Design review of the part built by this model. Coordinates are the model's own, in mm. A direction names the side the tool comes from. Round coordinates to 2 decimals unless told otherwise and drop trailing zeros. Order: outer loops, then holes, each group sorted by start corner. A loop starts at its lowest first (then second) coordinate and runs counter-clockwise, first axis right, second up. Notation, with made-up numbers: M 2.25,-25.5 L 53.25,-25.5 A13 cw 53.25,-21.5 Z; hole C -25,39 d8. An arc over 180 degrees is marked long. Use a Markdown table: item, result. Add a question column.
(1) Take a section at D-D (x = -2.75). Write out the cut boundary in (y, z), then the cut area to 3 significant figures.
(2) Take a section at A-A (z = -80.75). Write out the cut boundary in (x, y).
(3) The part is to be moulded in two halves that separate along X. For faces 1 (the face through (-0.212, -5.865, -82.733)), 2 (the face through (0, 3, -79.691)), 3 (the face through (5.18, 3.06, -82.73)), 4 (the face through (-6.454, -2.814, -94.712)), say which applies: released by +X, released by -X, zero draft, split by the parting line, or undercut.
(4) Take a section at C-C (x = 0). Write out the cut boundary in (y, z).
(5) For pin 1 (1 mm diameter, centred on x = -5.5, z = -92.5, fed in from +Y); pin 2 (1 mm diameter, centred on y = 1.5, z = -84.5, fed in from -X); pin 3 (6 mm diameter, centred on x = -3, z = -82.5, fed in from +Y), all flat-tipped, find the tip position at first contact; note any pin that passes through.
(6) Take a section at B-B (y = 0). Write out the cut boundary in (x, z), then the cut area to 3 significant figures.
(7) To check wall thickness, follow probe 1 along Z at (x, y) = (0.75, -8.5); probe 2 along Z at (x, y) = (-6.25, -0.75); probe 3 along Y at (x, z) = (5.25, -93.5). State the ranges of each line that lie inside material, in increasing order. Write a range as from..to.
(8) Machinability: for faces 5 (the face through (0.9, 2, -82.7)), 6 (the face through (3.94, -2.81, -94.71)), 7 (the face through (-0.2, -6.1, -85.691)), 8 (the face through (-0.018, 4.034, -82.733)), 9 (the face through (-3.408, -3.633, -91.959)), which of the approach directions +Z, -Z, +X, -X, +Y, -Y give a long, thin tool a straight path to every point of the face, cutting with its end or side? Answer none if there is none.
```python
from build123d import *

# Parameters (mm, degrees)
SKETCH2_R           = 10
SKETCH2_R_2         = 2.1
SKETCH2_R_3         = 1.2
BOSS_EXTRUDE1_DEPTH = 3
SKETCH3_R           = 10
SKETCH3_R_2         = 2
SKETCH3_R_3         = 2.1
BOSS_EXTRUDE2_DEPTH = 2.5
SKETCH4_R           = 2.1
BOSS_EXTRUDE3_DEPTH = 5
FILLET1_R           = 0.8
SKETCH5_R           = 2.1
BOSS_EXTRUDE4_DEPTH = 6


with BuildPart() as part:
    # Sketch2 → Boss-Extrude1 (new body)
    with BuildSketch(Plane.XY.offset(-96.191169136)):
        Circle(SKETCH2_R)
        Circle(SKETCH2_R_2, mode=Mode.SUBTRACT)
        with Locations((-0.05897353, 6.133133301)):
            Circle(SKETCH2_R_3, mode=Mode.SUBTRACT)
        with Locations((5.137178892, -2.866866699)):
            Circle(SKETCH2_R_3, mode=Mode.SUBTRACT)
        with Locations((-5.255125953, -2.866866699)):
            Circle(SKETCH2_R_3, mode=Mode.SUBTRACT)
    extrude(amount=BOSS_EXTRUDE1_DEPTH)

    # Sketch3 → Boss-Extrude2 (add)
    with BuildSketch(Plane.XY.offset(-93.191169136)):
        Circle(SKETCH3_R)
        with Locations((-5.255125953, -2.866866699)):
            Circle(SKETCH3_R_2, mode=Mode.SUBTRACT)
        with Locations((-0.05897353, 6.133133301)):
            Circle(SKETCH3_R_2, mode=Mode.SUBTRACT)
        with Locations((5.137178892, -2.866866699)):
            Circle(SKETCH3_R_2, mode=Mode.SUBTRACT)
        Circle(SKETCH3_R_3, mode=Mode.SUBTRACT)
    extrude(amount=BOSS_EXTRUDE2_DEPTH)

    # Sketch4 → Boss-Extrude3 (add)
    with BuildSketch(Plane.XY.offset(-90.691169136)):
        with BuildLine():
            ThreePointArc((7.264990173, -3.103210883), (6.783257612, 4.049372318), (0.715851765, 7.8675))
            ThreePointArc((0.715851765, 7.8675), (-0.040708899, 4.233646925), (-0.867006302, 7.852279928))
            ThreePointArc((-0.867006302, 7.852279928), (-6.879264147, 3.884034604), (-7.171380747, -3.313804186))
            ThreePointArc((-7.171380747, -3.313804186), (-3.527763738, -1.924526353), (-6.668183396, -4.236192889))
            ThreePointArc((-6.668183396, -4.236192889), (-0.191069364, -7.897689061), (6.455528982, -4.553695814))
            ThreePointArc((6.455528982, -4.553695814), (3.267691347, -1.823575878), (7.264990173, -3.103210883))
        make_face()
        Circle(SKETCH4_R, mode=Mode.SUBTRACT)
    extrude(amount=BOSS_EXTRUDE3_DEPTH)

    # Fillet1
    # the kernel refuses this fillet: 0.8 mm, written as the material it takes off along each edge
    with BuildSketch(Plane(origin=(-0.867006302, 7.852279928, -90.691169136), x_dir=(-0.9684268820768696, -0.24929776186494912, 0), z_dir=(0, 0, 1))) as fillet1_piece_1:
        with BuildLine():
            CenterArc((2.122639751, 0.791949539), FILLET1_R, 156.548445833, 121.586747485)
            ThreePointArc((1.388722227, 1.110328352), (0.832290223, 0.382651946), (0, 0))
            ThreePointArc((0, 0), (1.117923602, -0.079498301), (2.235847204, 0))
        make_face()
    extrude(amount=10.589618011, mode=Mode.SUBTRACT)
    with BuildSketch(Plane(origin=(-7.171380747, -3.313804186, -90.691169136), x_dir=(-0.2672810953743128, 0.9636186050795758, 0), z_dir=(0, 0, 1))) as fillet1_piece_2:
        with BuildLine():
            CenterArc((2.423675061, -0.789487911), FILLET1_R, 80.701479552, 124.454730774)
            ThreePointArc((1.699553301, -1.129558017), (1.007651544, -0.327237606), (0, 0))
            ThreePointArc((0, 0), (1.276468866, 0.103806875), (2.552937731, 0))
        make_face()
    extrude(amount=11.382344328, mode=Mode.SUBTRACT)
    with BuildSketch(Plane(origin=(-6.668183396, -4.236192889, -90.691169136), x_dir=(0.9674204056157966, -0.2531753518772465, 0), z_dir=(0, 0, 1))) as fillet1_piece_3:
        with BuildLine():
            CenterArc((2.455521009, -0.684038404), FILLET1_R, 121.234961486, 124.454730774)
            ThreePointArc((2.126178356, -1.413101787), (1.005630009, -0.793004992), (0, 0))
            ThreePointArc((0, 0), (1.020340965, -0.285219915), (2.040681929, 0))
        make_face()
    extrude(amount=11.382344328, mode=Mode.SUBTRACT)
    with BuildSketch(Plane(origin=(6.455528982, -4.553695814, -90.691169136), x_dir=(-0.9836137954546407, -0.18028838396113095, 0), z_dir=(0, 0, 1))) as fillet1_piece_4:
        with BuildLine():
            CenterArc((2.356185075, 0.708813813), FILLET1_R, 116.541300521, 125.835667041)
            ThreePointArc((1.998710841, 1.42450381), (0.943696464, 0.790346579), (0, 0))
            ThreePointArc((0, 0), (0.99263164, 0.244025278), (1.98526328, 0))
        make_face()
    extrude(amount=11.13598817, mode=Mode.SUBTRACT)
    with BuildSketch(Plane(origin=(7.264990173, -3.103210883, -90.691169136), x_dir=(0.2451881288110309, 0.969475518767826, 0), z_dir=(0, 0, 1))) as fillet1_piece_5:
        with BuildLine():
            CenterArc((2.33012209, 0.790288667), FILLET1_R, 153.100934038, 125.835667041)
            ThreePointArc((1.616678166, 1.152224804), (0.94996865, 0.377392996), (0, 0))
            ThreePointArc((0, 0), (1.227197634, -0.095899413), (2.454395268, 0))
        make_face()
    extrude(amount=11.13598817, mode=Mode.SUBTRACT)
    with BuildSketch(Plane(origin=(0.715851765, 7.8675, -90.691169136), x_dir=(0.6159695110319643, -0.7877699927510841, 0), z_dir=(0, 0, 1))) as fillet1_piece_6:
        with BuildLine():
            CenterArc((2.152431859, 0.70697997), FILLET1_R, 120.508273334, 121.586747485)
            ThreePointArc((1.746301639, 1.396224661), (0.823506332, 0.760204236), (0, 0))
            ThreePointArc((0, 0), (0.889013284, 0.22087306), (1.778026567, 0))
        make_face()
    extrude(amount=10.589618011, mode=Mode.SUBTRACT)

    # Sketch5 → Boss-Extrude4 (add)
    with BuildSketch(Plane.XY.offset(-85.691169136)):
        with BuildLine():
            ThreePointArc((5.84214559, -0.951667659), (5.152070119, 3.107191821), (2.00838279, 5.765720437))
            ThreePointArc((2.00838279, 5.765720437), (-0.05897353, 4.033382276), (-2.126329851, 5.765720437))
            ThreePointArc((-2.126329851, 5.765720437), (-5.315006226, 3.026940535), (-5.924054987, -1.132101661))
            ThreePointArc((-5.924054987, -1.132101661), (-3.644953029, -1.937232928), (-4.087239877, -4.313558756))
            ThreePointArc((-4.087239877, -4.313558756), (-0.150972365, -5.866161342), (3.831051219, -4.434985289))
            ThreePointArc((3.831051219, -4.434985289), (3.369772867, -1.846454355), (5.84214559, -0.951667659))
        make_face()
        with Locations(Location((-0.05897353, 0.133133301, 0), (0, 0, 205.878507887))):
            Circle(SKETCH5_R, mode=Mode.SUBTRACT)
    extrude(amount=BOSS_EXTRUDE4_DEPTH)


solid = part.part
```
Verdict:
| question | item | result |
|---|---|---|
| 1 | outline | M -9.61,-96.19 L 9.61,-96.19 L 9.61,-90.69 L 7.36,-90.69 L 7.36,-85.69 L 5.5,-85.69 L 5.5,-79.69 L -5.23,-79.69 L -5.23,-85.69 L -7.41,-85.69 L -7.41,-90.69 L -9.61,-90.69 Z |
| 1 | area | 244 mm^2 |
| 2 | outline | M -5.92,-1.13 A1.86 cw -4.09,-4.31 A6 ccw 3.83,-4.43 A2.04 cw 5.84,-0.95 A6 ccw 2.01,5.77 A2.1 cw -2.13,5.77 A6 ccw Z; hole C -0.06,0.13 d4.2 |
| 3 | face 1 | split by the parting line |
| 3 | face 2 | zero draft |
| 3 | face 3 | released by +X |
| 3 | face 4 | undercut |
| 4 | outline | M -10,-96.19 L -2.1,-96.19 L -2.1,-85.69 L -1.97,-85.69 L -1.97,-79.69 L -5.87,-79.69 L -5.87,-85.69 L -7.9,-85.69 L -7.9,-90.69 L -10,-90.69 Z; M 2.1,-96.19 L 4.93,-96.19 L 4.93,-93.19 L 4.13,-93.19 L 4.13,-90.69 L 4.23,-90.69 L 4.23,-85.69 L 4.03,-85.69 L 4.03,-79.69 L 2.23,-79.69 L 2.23,-85.69 L 2.1,-85.69 Z; M 7.33,-96.19 L 10,-96.19 L 10,-90.69 L 8.13,-90.69 L 8.13,-93.19 L 7.33,-93.19 Z |
| 5 | pin 1 | stops at y = 8.66 |
| 5 | pin 2 | stops at x = -6 |
| 5 | pin 3 | stops at y = 5.77 |
| 6 | outline | M -10,-96.19 L -2.1,-96.19 L -2.1,-85.69 L -2.15,-85.69 L -2.15,-79.69 L -6.06,-79.69 L -6.06,-85.69 L -7.9,-85.69 L -7.9,-90.69 L -10,-90.69 Z; M 2.04,-85.69 L 2.1,-85.69 L 2.1,-96.19 L 10,-96.19 L 10,-90.69 L 7.9,-90.69 L 7.9,-85.69 L 5.94,-85.69 L 5.94,-79.69 L 2.04,-79.69 Z |
| 6 | area | 192 mm^2 |
| 7 | probe 1 | z = -96.19..-90.69 |
| 7 | probe 2 | z = -96.19..-85.69 |
| 7 | probe 3 | y = -8.51..-4.06, -1.67..8.51 |
| 8 | face 5 | +Z |
| 8 | face 6 | +Z, -Z |
| 8 | face 7 | +Z, -Y |
| 8 | face 8 | +Z, +Y |
| 8 | face 9 | none |
